from build123d import *

# Parameters (mm, degrees)
PAD_DEPTH            = 90
POCKET_DEPTH         = 4
BODY_PLACEMENT_ANGLE = 90


with BuildPart() as part:
    # Sketch → Pad (new body)
    with BuildSketch(Plane.XY):
        Polygon((0, 29.646015), (-30.420355, 0), (-30.420355, -40.486725), (30.420351, -40.486725), (30.420351, 0), align=None)
    extrude(amount=PAD_DEPTH)

    # Sketch001 (on Face7 of Pad) → Pocket (cut)
    with BuildSketch(Plane.XY.offset(90)):
        Polygon((-19.370302, -13.946699), (-19.370302, -40.940281), (-4.869621, -40.940281), (-4.869621, -14.615959), align=None)
        Polygon((8.111094, -5.154654), (8.659041, -12.825894), (12.859957, -12.460593), (12.312009, -5.337305), align=None)
        Polygon((14.138495, -5.337304), (14.138495, -13.008539), (18.52206, -12.825896), (18.704708, -6.067894), align=None)
        Polygon((8.476391, -13.921784), (12.677306, -13.921784), (13.225254, -21.045074), (7.745796, -21.045074), align=None)
        Polygon((14.138495, -14.469728), (15.05174, -21.410372), (18.887358, -21.593025), (18.887358, -14.469728), align=None)
        Polygon((-26.966421, 0), (0.250248, 26.098402), (26.797653, 0), align=None)
    extrude(amount=-POCKET_DEPTH, mode=Mode.SUBTRACT)


with BuildPart() as part_1:
    # Body placement: moved
    add(part.part.rotate(Axis((0, 0, 0), (1, 0, 0)), BODY_PLACEMENT_ANGLE))


solid = part_1.part
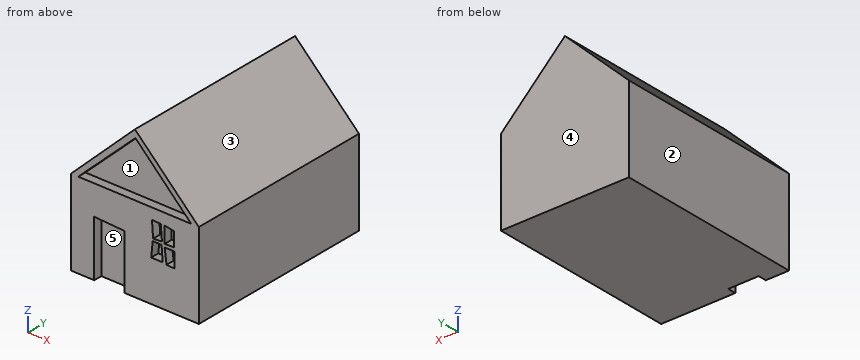
Geometry: final body of the model. Coordinates: model frame, mm. Face numbers are marked on the shaded views. A direction names the side the tool comes from. Round coordinates to 2 decimals unless told otherwise and drop trailing zeros. Loops run counter-clockwise (first coordinate to the right, second up) from the corner with the lowest first, then second, coordinate; pieces in that order, holes last.
Q1. Section A-A on z = 17.5. Return loops of the section in (x, y), plus the area to 3 significant figures.
Q2. Access query for the marked faces 4 and 5. Directions: +Z, -Z, +X, -X, +Y, -Y. A direction counts if a zero-diameter tool reaches every point of the face in a straight line with its end or side. Return the directions, or none.
Q3. Section D-D on z = -20. Return loops of the section in (x, y), plus the area to 3 significant figures.
Q4. Section C-C on x = 3.5. Return loops of the section in (y, z), plus the area to 3 significant figures.
Q5. Material intervals for L1, parallel to Y at x = -7, z = -35.5; L2, parallel to Z at x = -15, y = -49.5; L3, parallel to X at y = -24.5, z = 6.5, sorted ascending.
Q6. Pull-direction query (Z, two-part tool) for the marked faces 1, 2 and 3; classes: released by +Z, released by -Z, zero draft, split by the parting line, or undercut.
Q7. Pin query (flat end, axial travel): P1, Ø3, axis at x = 10.5, y = -87.5, coming from the +Z side; P2, Ø13, axis at x = -4, z = 7, coming from the -Y side; P3, Ø1.2, axis at x = -4.5, y = -88.5, coming from the +Z side. Return the tip coordinate at first contact, or that it passes through.
Q8. Section B-B on y = -63.5. Return loops of the section in (x, z), plus the area to 3 significant figures.
Evaluation:
1. outline: (-12.46, -90) - (-8.72, -90) - (-8.72, -86) - (9, -86) - (9, -90) - (12.46, -90) - (12.46, 0) - (-12.46, 0) - close
1. area: 2,170 mm2
2. face 4: +Z, -Z, +X, -X, +Y
2. face 5: -Z, -Y
3. outline: (-30.42, -90) - (-19.37, -90) - (-19.37, -86) - (-4.87, -86) - (-4.87, -90) - (7.85, -90) - (7.85, -86) - (13.14, -86) - (13.14, -90) - (14.87, -90) - (14.87, -86) - (18.89, -86) - (18.89, -90) - (30.42, -90) - (30.42, 0) - (-30.42, 0) - close
3. area: 5,380 mm2
4. outline: (-90, -40.49) - (0, -40.49) - (0, 26.24) - (-90, 26.24) - (-90, 22.9) - (-86, 22.9) - (-86, 0) - (-90, 0) - close
4. area: 5,910 mm2
5. L1: y = -86 to 0
5. L2: z = -40.49 to 15.03
5. L3: x = -23.75 to 23.75
6. face 1: undercut
6. face 2: zero draft
6. face 3: released by +Z
7. P1: stops at z = 20.88
7. P2: stops at y = -86
7. P3: stops at z = 25.85
8. outline: (-30.42, -40.49) - (30.42, -40.49) - (30.42, 0) - (0, 29.65) - (-30.42, 0) - close
8. area: 3,370 mm2
